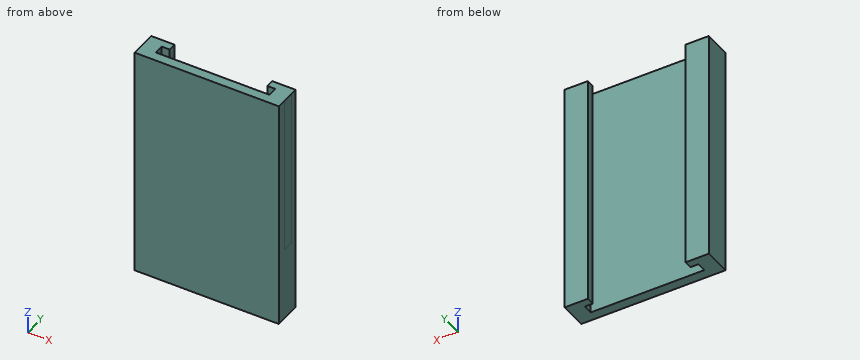
Autodesk Inventor part; units mm, degrees
ref_plane "YZ Plane" through (0, 0, 0) normal (1, 0, 0) x (0, 1, 0)
ref_plane "XZ Plane" through (0, 0, 0) normal (0, 1, 0) x (-1, 0, 0)
ref_plane "XY Plane" through (0, 0, 0) normal (0, 0, 1) x (1, 0, 0)
sketch "Sketch1" plane through (0, 0, 0) normal (0, 1, 0) x (-1, 0, 0)
  line L0 (-32.5, 25) -> (32.5, 25)
  line L1 (32.5, 25) -> (32.5, -25)
  line L2 (32.5, -25) -> (-32.5, -25)
  line L3 (-32.5, -25) -> (-32.5, 25)
  line L4 (-32.5, 25) -> (32.5, -25) construction
  line L5 (32.5, 25) -> (-32.5, -25) construction
  point P0 (0, 0)
  dimension "d0" = 65
  dimension "d1" = 50
extrude "Extrusion1" add sketch "Sketch1" along normal blind 3
sketch "Sketch2" plane through (0, 3, 0) normal (0, 1, 0) x (1, 0, 0)
  line L0 (32.5, 25) -> (-32.5, 25)
  line L1 (-18.25, -25) -> (18.25, -25)
  line L2 (18.25, -25) -> (18.25, 25)
  line L3 (18.25, 25) -> (-18.25, 25)
  line L4 (-18.25, 25) -> (-18.25, -25)
  line L5 (-18.25, -25) -> (18.25, 25) construction
  line L6 (18.25, -25) -> (-18.25, 25) construction
  line L7 (-22.5, -25) -> (22.5, -25)
  line L8 (22.5, -25) -> (22.5, 25)
  line L9 (22.5, 25) -> (-22.5, 25)
  line L10 (-22.5, 25) -> (-22.5, -25)
  line L11 (-22.5, -25) -> (22.5, 25) construction
  line L12 (22.5, -25) -> (-22.5, 25) construction
  point P0 (0, 0)
  dimension "d4" = 36.5
  dimension "d5" = 45
extrude "Extrusion2" add sketch "Sketch2" along normal blind 3.5 contours L8 L7 L2 L0 | L4 L7 L10 L0
sketch "Sketch3" plane through (0, 6.5, 0) normal (0, 1, 0) x (1, 0, 0)
  line L0 (-22.5, 25) -> (-32.5, 25)
  line L1 (-22.5, 25) -> (-15.25, 25)
  line L2 (-15.25, 25) -> (-15.25, -25)
  line L3 (-15.25, -25) -> (-22.5, -25)
  line L4 (-22.5, -25) -> (-22.5, 25)
  line L5 (-32.5, -25) -> (32.5, -25)
  line L6 (32.5, 25) -> (-32.5, 25)
  line L7 (22.4999, -25) -> (15.2499, -25)
  line L8 (15.2499, -25) -> (15.2499, 25)
  line L9 (15.2499, 25) -> (22.4999, 25)
  line L10 (22.4999, 25) -> (22.4999, -25)
  point P0 (0, 0)
  dimension "d8" = 7.25
  dimension "d9" = 7.25
extrude "Extrusion3" add sketch "Sketch3" along normal blind 2 contours L1 L2 L3 L4 | L6 L10 L5 L8
sketch "Sketch4" plane through (0, 3, 0) normal (0, 1, 0) x (1, 0, 0)
  line L0 (-22.5, 25) -> (-22.5, -25)
  line L1 (-32.5, 25) -> (-32.5, -25)
  line L2 (-22.5, 25) -> (-32.5, 25)
  line L3 (-32.5, 25) -> (-32.5, -25)
  line L4 (-32.5, -25) -> (-22.5, -25)
  line L5 (-22.5, -25) -> (-22.5, 25)
  line L6 (22.4999, -25) -> (22.4999, 25)
  line L7 (-32.5, -25) -> (32.5, -25)
  line L8 (22.4999, 25) -> (32.5, 25)
  line L9 (32.5, 25) -> (32.5, -25)
  line L10 (32.5, -25) -> (22.4999, -25)
  line L11 (22.4999, -25) -> (22.4999, 25)
  point P0 (0, 0)
extrude "Extrusion4" cut sketch "Sketch4" against normal blind 10
sketch "Sketch5" plane through (-18.25, 3, 25) normal (1, 0, 0) x (0, 0, -1)
  line L0 (0, 3.5) -> (50, 3.5)
  line L1 (50, 0) -> (0, 0)
  line L2 (0, 0) -> (0, 3.5)
  line L3 (0, 3.5) -> (50, 3.5)
  line L4 (50, 3.5) -> (50, 0)
  point P0 (25, -3)
extrude "Extrusion5" add sketch "Sketch5" along normal blind 0.5
sketch "Sketch6" plane through (18.25, 3, -25) normal (-1, 0, 0) x (0, 0, 1)
  line L0 (50, 0) -> (50, 3.5)
  line L1 (0, 0) -> (0, -3)
  line L2 (50, 3.5) -> (0, 3.5)
  line L3 (0, 3.5) -> (0, 0)
  line L4 (0, 0) -> (50, 0)
  line L5 (50, 0) -> (50, 3.5)
  point P0 (25, -3)
extrude "Extrusion6" add sketch "Sketch6" along normal blind 0.5
sketch "Sketch7" plane through (0, 6.5, 0) normal (0, -1, 0) x (1, 0, 0)
  line L0 (15.2499, 25) -> (17.75, 25)
  line L1 (15.2499, -25) -> (17.75, -25)
  line L2 (17.75, -25) -> (17.75, 25)
  line L3 (17.75, 25) -> (15.2499, 25)
  line L4 (15.2499, 25) -> (15.2499, -25)
  line L5 (-15.25, 25) -> (-17.75, 25)
  line L6 (-17.75, 25) -> (-17.75, -25)
  line L7 (-17.75, -25) -> (-15.25, -25)
  line L8 (-15.25, -25) -> (-15.25, 25)
  point P0 (0, 0)
extrude "Extrusion7" add sketch "Sketch7" along normal blind 0.5
sketch "Sketch8" plane through (-15.25, 8.5, -25) normal (0, 0, -1) x (-1, 0, 0)
  line L0 (0, -2.5) -> (0, 0)
  line L1 (0, -2.5) -> (0, 0)
  line L2 (7.25, 0) -> (0, 0)
  line L3 (0, 0) -> (7.25, 0)
  line L4 (7.25, 0) -> (7.25, -8.5)
  line L5 (7.25, 0) -> (7.25, -8.5)
  line L6 (7.25, -8.5) -> (-37.7499, -8.5)
  line L7 (7.25, -8.5) -> (-37.7499, -8.5)
  line L8 (-37.7499, -2) -> (-37.7499, 0)
  line L9 (-37.7499, -8.5) -> (-37.7499, 0)
  line L10 (-37.7499, 0) -> (-30.4999, 0)
  line L11 (-37.7499, 0) -> (-30.4999, 0)
  line L12 (-30.4999, -2.5) -> (-30.4999, 0)
  line L13 (-30.4999, 0) -> (-30.4999, -2.5)
  line L14 (-30.4999, -2.5) -> (-33, -2.5)
  line L15 (-33, -5.5) -> (-33, -2.5)
  line L16 (-33, -2.5) -> (-33, -5.5)
  line L17 (-33, -5.5) -> (2.5, -5.5)
  line L18 (-33, -5.5) -> (2.5, -5.5)
  line L19 (2.5, -2.5) -> (2.5, -5.5)
  line L20 (2.5, -5.5) -> (2.5, -2.5)
  line L21 (0, -2.5) -> (2.5, -2.5)
  line L22 (2.5, -2.5) -> (0, -2.5)
  point P0 (-15.25, -8.5)
extrude "Extrusion8" add sketch "Sketch8" along normal blind 23
properties part number "DINsupport"
Source: CAD feature listing. Evaluate the final solid. Frame: model axes, mm. Round coordinates to 2 decimals unless told otherwise and drop trailing zeros. Loops run counter-clockwise (first coordinate to the right, second up) from the corner with the lowest first, then second, coordinate; pieces in that order, holes last. Notation, with made-up numbers: (58, 79.5) -> (98, 79.5) arc R23 ccw to (98, 99.5) -> close; hole circle Ø10 at (-15.5, 77.25). An arc over 180 degrees is marked (long way). Answer as a JSON object with one key per item and string values. Group by question number.
Q1. Ray query, line 1 (X direction, y = 5.25, z = -37.5); line 2 (X direction, y = 7, z = -3); line 3 (Y direction, x = -7.5, z = -5.5). Return the intervals inside material, ascending. Write a range as from..to.
Q2. Section query B-B (x = -16). Output: boundary loops of the cut face in (y, z).
Q3. Section query A-A (y = 7.75). Output: boundary loops of the cut face in (x, z), plus the area to 3 significant figures.
Q4. Contact query for a flat-ended pin moving along its axis: P1, Ø5, axis at x = -12, y = 7, coming from the -Z side. Output: stop coordinate, or through.
Completed:
{
 "1": {"line 1": "-22.5..-17.75, 17.75..22.5", "line 2": "-22.5..-15.25, 15.25..22.5", "line 3": "0..3"},
 "2": {"outline": "(0, -48) -> (3, -48) -> (3, 25) -> (0, 25) -> close; (6, -48) -> (8.5, -48) -> (8.5, 25) -> (6, 25) -> close"},
 "3": {"outline": "(-22.5, -48) -> (-15.25, -48) -> (-15.25, 25) -> (-22.5, 25) -> close; (15.25, -48) -> (22.5, -48) -> (22.5, 25) -> (15.25, 25) -> close", "area": "1,060 mm²"},
 "4": {"P1": "through"}
}
